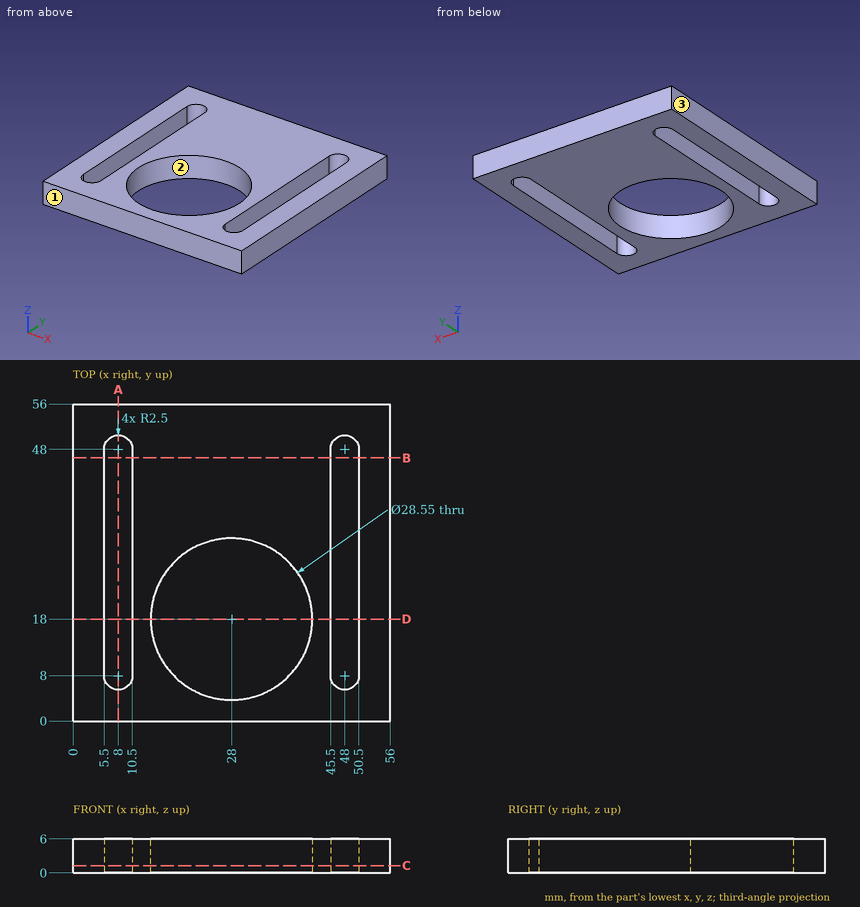
Job drawing, mm, ordinate dimensions from the low corner. One solid piece. Round coordinates to 2 decimals unless told otherwise and drop trailing zeros. Loops run counter-clockwise (first coordinate to the right, second up) from the corner with the lowest first, then second, coordinate; pieces in that order, holes last. Notation, with made-up numbers: (65, -4) -> (122, -4) arc R25 ccw to (122, 32) -> close; hole circle Ø7 at (64, 83). An arc over 180 degrees is marked (long way). One line per item, written item: value. Start each with the question number.
Q1. Cut at A-A on x = 8. List the corners of the cut face in (y, z), plus the area to 3 significant figures.
Q2. Cut at C-C on z = 1.3. List the corners of the cut face in (x, y) (3 decimals).
Q3. Cut at B-B on y = 46.5. List the corners of the cut face in (x, z), plus the area to 3 significant figures.
Q4. Cut at D-D on y = 18. List the corners of the cut face in (x, z) (3 decimals), plus the area to 3 significant figures.
Q5. Probe line 1 along X through (y, z) = (34, 4.05); line 2 along Y through (x, z) = (28, 1.4) (3 decimals); line 3 along X through (y, z) = (13, 1.1). List the from-to ranges inside material, lowest first.
Q6. Two-plate mould, pull along X, no slides. Class the marked faces 1, 2 and 3: released by +X, released by -X, zero draft, split by the parting line, or undercut.
Q7. Drop a flat-ended pin along its axis: pin 1 Ø3 at (x, z) = (36, 5) entering from -Y. Give the stop position or say it passes through.
Computed:
1. outline: (0, 0) -> (5.5, 0) -> (5.5, 6) -> (0, 6) -> close; (50.5, 0) -> (56, 0) -> (56, 6) -> (50.5, 6) -> close
1. area: 66.0 mm²
2. outline: (0, 0) -> (56, 0) -> (56, 56) -> (0, 56) -> close; hole (5.5, 8) arc R2.5 ccw to (10.5, 8) -> (10.5, 48) arc R2.5 ccw to (5.5, 48) -> close; hole circle Ø28.55 at (28, 18); hole (45.5, 8) arc R2.5 ccw to (50.5, 8) -> (50.5, 48) arc R2.5 ccw to (45.5, 48) -> close
3. outline: (0, 0) -> (5.5, 0) -> (5.5, 6) -> (0, 6) -> close; (10.5, 0) -> (45.5, 0) -> (45.5, 6) -> (10.5, 6) -> close; (50.5, 0) -> (56, 0) -> (56, 6) -> (50.5, 6) -> close
3. area: 276 mm²
4. outline: (0, 0) -> (5.5, 0) -> (5.5, 6) -> (0, 6) -> close; (10.5, 0) -> (13.725, 0) -> (13.725, 6) -> (10.5, 6) -> close; (42.275, 0) -> (45.5, 0) -> (45.5, 6) -> (42.275, 6) -> close; (50.5, 0) -> (56, 0) -> (56, 6) -> (50.5, 6) -> close
4. area: 105 mm²
5. line 1: 0 to 5.5, 10.5 to 45.5, 50.5 to 56
5. line 2: 0 to 3.725, 32.275 to 56
5. line 3: 0 to 5.5, 10.5 to 14.63, 41.37 to 45.5, 50.5 to 56
6. face 1: zero draft
6. face 2: undercut
6. face 3: released by -X
7. pin 1: y = 0
